Input: dimensioned drawing with shaded views. Units: mm. Origin: part minimum x, y, z. Coordinates: 2 decimals unless noted, no trailing zeros. Order: outer loops, then holes, each group sorted by start corner. A loop starts at its lowest first (then second) coordinate and runs counter-clockwise, first axis right, second up. Notation, with made-up numbers: (69.5, 6.25) -> (104.5, 6.25) arc R15 cw to (104.5, 16.25) -> close; hole circle Ø6 at (-40, 7). An arc over 180 degrees is marked (long way). Put each result on its own line as item: value.
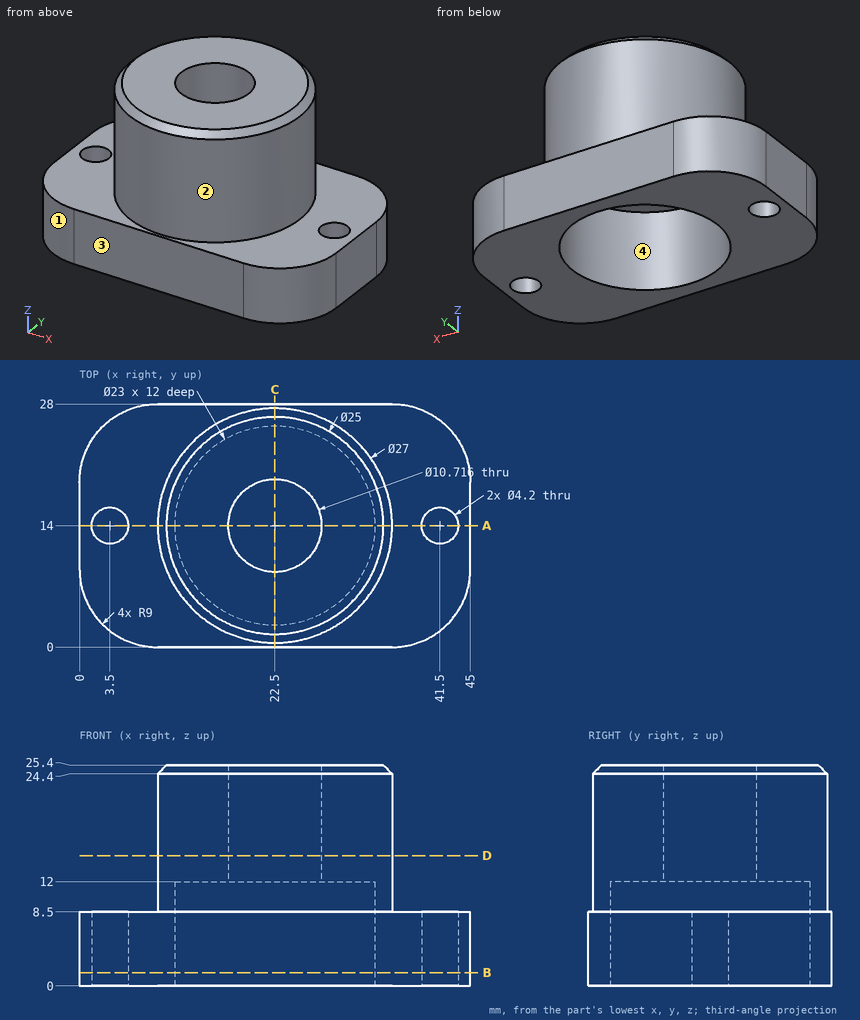
1. Ray query, line 1 along X through (y, z) = (13.75, 10); line 2 along Y through (x, z) = (22.5, 6.5); line 3 along Y through (x, z) = (22.5, 15). Return the intervals inside material, ascending.
Numbers:
line 1: x = 9 to 11, 34 to 36
line 2: y = 0 to 2.5, 25.5 to 28
line 3: y = 0.5 to 8.64, 19.36 to 27.5
2. Cut plane B-B on z = 1.5. Output: boundary loops of the cut face in (x, y).
Numbers:
outline: (0, 9) arc R9 ccw to (9, 0) -> (36, 0) arc R9 ccw to (45, 9) -> (45, 19) arc R9 ccw to (36, 28) -> (9, 28) arc R9 ccw to (0, 19) -> close; hole circle Ø4.2 at (3.5, 14); hole circle Ø23 at (22.5, 14); hole circle Ø4.2 at (41.5, 14)
3. Cut plane D-D on z = 15. Output: boundary loops of the cut face in (x, y), plus the area to 3 significant figures.
Numbers:
outline: circle Ø27 at (22.5, 14); hole circle Ø10.72 at (22.5, 14)
area: 482 mm2
4. Cut plane C-C on x = 22.5. Output: boundary loops of the cut face in (y, z), plus the area to 3 significant figures.
Numbers:
outline: (0, 0) -> (2.5, 0) -> (2.5, 12) -> (8.64, 12) -> (8.64, 25.4) -> (1.5, 25.4) -> (0.5, 24.4) -> (0.5, 8.5) -> (0, 8.5) -> close; (19.36, 12) -> (25.5, 12) -> (25.5, 0) -> (28, 0) -> (28, 8.5) -> (27.5, 8.5) -> (27.5, 24.4) -> (26.5, 25.4) -> (19.36, 25.4) -> close
area: 274 mm2
5. Cut plane A-A on y = 14. Output: boundary loops of the cut face in (x, z), plus the area to 3 significant figures.
Numbers:
outline: (0, 0) -> (1.4, 0) -> (1.4, 8.5) -> (0, 8.5) -> close; (5.6, 0) -> (11, 0) -> (11, 12) -> (17.14, 12) -> (17.14, 25.4) -> (10, 25.4) -> (9, 24.4) -> (9, 8.5) -> (5.6, 8.5) -> close; (27.86, 12) -> (34, 12) -> (34, 0) -> (39.4, 0) -> (39.4, 8.5) -> (36, 8.5) -> (36, 24.4) -> (35, 25.4) -> (27.86, 25.4) -> close; (43.6, 0) -> (45, 0) -> (45, 8.5) -> (43.6, 8.5) -> close
area: 347 mm2
6. First-contact query: pin 1 (4 mm diameter, centred on x = 16.5, z = 17.5, fed in from -Y); pin 2 (1.5 mm diameter, centred on x = 29.5, z = 17, fed in from -Y); pin 3 (4 mm diameter, centred on x = 6.5, z = 7, fed in from +Y); pin 4 (4 mm diameter, centred on x = 41.5, y = 14, fed in from -Z). Flat tips, straight axial feed; report the tip coordinate or a pass-through.
Numbers:
pin 1: stops at y = 1.11
pin 2: stops at y = 2.03
pin 3: stops at y = 27.99
pin 4: passes through
7. Pull-direction query (X, two-part tool) for the marked faces 1, 2, 3 and 4; classes: pulls with the +X half, pulls with the -X half, needs draft (parallel to the pull), parting line crosses it, or undercut.
Numbers:
face 1: pulls with the -X half
face 2: parting line crosses it
face 3: needs draft
face 4: undercut
